The listing builds one solid part. Answer for the finished solid, in the listing's coordinates (mm). A direction names the side the tool comes from. Coordinates: 2 decimals unless noted, no trailing zeros. Order: outer loops, then holes, each group sorted by start corner. A loop starts at its lowest first (then second) coordinate and runs counter-clockwise, first axis right, second up.
```python
from build123d import *

# Parameters (mm, degrees)
BOSS_EXTRUDE1_DEPTH = 25
SKETCH2_R           = 11.025
CUT_EXTRUDE1_DEPTH  = 7
CUT_EXTRUDE3_DEPTH  = 8.75
CUT_EXTRUDE5_DEPTH  = 8.75
SKETCH5_R           = 1
CUT_EXTRUDE6_DEPTH  = 7.5
SKETCH6_R           = 1.95
CUT_EXTRUDE7_DEPTH  = 6.5
SKETCH7_R           = 2
CUT_EXTRUDE8_DEPTH  = 1
CUT_EXTRUDE9_DEPTH  = 62.065538563
CUT_EXTRUDE10_DEPTH = 3.5
SKETCH10_W          = 40
SKETCH10_H          = 5.05
CUT_EXTRUDE11_DEPTH = 7


with BuildPart() as part:
    # Sketch1 → Boss-Extrude1 (new body)
    with BuildSketch(Plane(origin=(0, 0, 0), x_dir=(1, 0, 0), z_dir=(0, 1, 0))):
        with BuildLine():
            Line((-42, -10), (42, -10))
            ThreePointArc((42, -10), (52, 0), (42, 10))
            Line((42, 10), (-42, 10))
            ThreePointArc((-42, 10), (-52, 0), (-42, -10))
        make_face()
    extrude(amount=BOSS_EXTRUDE1_DEPTH)

    # Sketch2 → Cut-Extrude1 (cut)
    with BuildSketch(Plane.XY.offset(10)):
        with Locations((0, 12.5)):
            Circle(SKETCH2_R)
    extrude(amount=-CUT_EXTRUDE1_DEPTH, mode=Mode.SUBTRACT)

    # Sketch3 → Cut-Extrude3 (cut)
    with BuildSketch(Plane.XZ):
        with BuildLine():
            Line((15, -10), (15, 10))
            Line((15, 10), (42, 10))
            ThreePointArc((42, 10), (52, 0), (42, -10))
            Line((42, -10), (15, -10))
        make_face()
        with BuildLine():
            Line((-15, -10), (-15, 10))
            Line((-15, 10), (-42, 10))
            ThreePointArc((-42, 10), (-52, 0), (-42, -10))
            Line((-42, -10), (-15, -10))
        make_face()
    extrude(amount=-CUT_EXTRUDE3_DEPTH, mode=Mode.SUBTRACT)

    # Sketch4 → Cut-Extrude5 (cut)
    with BuildSketch(Plane(origin=(0, 25, 0), x_dir=(1, 0, 0), z_dir=(0, 1, 0))):
        with BuildLine():
            Line((15, -10), (15, 10))
            Line((15, 10), (55, 10))
            ThreePointArc((55, 10), (65, 0), (55, -10))
            Line((55, -10), (15, -10))
        make_face()
        with BuildLine():
            Line((-15, -10), (-15, 10))
            Line((-15, 10), (-55, 10))
            ThreePointArc((-55, 10), (-65, 0), (-55, -10))
            Line((-55, -10), (-15, -10))
        make_face()
    extrude(amount=-CUT_EXTRUDE5_DEPTH, mode=Mode.SUBTRACT)

    # Sketch5 → Cut-Extrude6 (cut)
    with BuildSketch(Plane(origin=(0, 16.25, 0), x_dir=(1, 0, 0), z_dir=(0, 1, 0))):
        with Locations(Location((-42, 6.2, 0), (0, 0, 270))):
            Circle(SKETCH5_R)
        with Locations(Location((-35.8, 0, 0), (0, 0, 270))):
            Circle(SKETCH5_R)
        with Locations(Location((-42, -6.2, 0), (0, 0, 270))):
            Circle(SKETCH5_R)
        with Locations(Location((-48.2, 0, 0), (0, 0, 270))):
            Circle(SKETCH5_R)
        with Locations(Location((42, 6.2, 0), (0, 0, 270))):
            Circle(SKETCH5_R)
        with Locations(Location((48.2, 0, 0), (0, 0, 270))):
            Circle(SKETCH5_R)
        with Locations(Location((42, -6.2, 0), (0, 0, 270))):
            Circle(SKETCH5_R)
        with Locations(Location((35.8, 0, 0), (0, 0, 270))):
            Circle(SKETCH5_R)
    extrude(amount=-CUT_EXTRUDE6_DEPTH, mode=Mode.SUBTRACT)

    # Sketch6 → Cut-Extrude7 (cut)
    with BuildSketch(Plane.XZ.offset(-8.75)):
        with Locations(Location((-42, 6.2, 0), (0, 0, 270))):
            Circle(SKETCH6_R)
        with Locations(Location((-35.8, 0, 0), (0, 0, 270))):
            Circle(SKETCH6_R)
        with Locations(Location((-48.2, 0, 0), (0, 0, 270))):
            Circle(SKETCH6_R)
        with Locations(Location((-42, -6.2, 0), (0, 0, 270))):
            Circle(SKETCH6_R)
        with Locations(Location((42, 6.2, 0), (0, 0, 270))):
            Circle(SKETCH6_R)
        with Locations(Location((48.2, 0, 0), (0, 0, 270))):
            Circle(SKETCH6_R)
        with Locations(Location((35.8, 0, 0), (0, 0, 270))):
            Circle(SKETCH6_R)
        with Locations(Location((42, -6.2, 0), (0, 0, 270))):
            Circle(SKETCH6_R)
    extrude(amount=-CUT_EXTRUDE7_DEPTH, mode=Mode.SUBTRACT)

    # Sketch7 → Cut-Extrude8 (cut)
    with BuildSketch(Plane(origin=(0, 16.25, 0), x_dir=(1, 0, 0), z_dir=(0, 1, 0))):
        with Locations(Location((-42, 0, 0), (0, 0, 270))):
            Circle(SKETCH7_R)
        with Locations(Location((42, 0, 0), (0, 0, 270))):
            Circle(SKETCH7_R)
    extrude(amount=-CUT_EXTRUDE8_DEPTH, mode=Mode.SUBTRACT)

    # Sketch8 → Cut-Extrude9 (cut, through all)
    with BuildSketch(Plane.XY.offset(10)):
        with BuildLine():
            Line((-15, 16.25), (-15, 25))
            Line((-15, 25), (-9.100137362, 25))
            ThreePointArc((-9.100137362, 25), (-12.819702813, 21.143941218), (-15, 16.25))
        make_face()
        with BuildLine():
            Line((15, 0), (9.100137362, 0))
            ThreePointArc((9.100137362, 0), (12.819702813, 3.856058782), (15, 8.75))
            Line((15, 8.75), (15, 0))
        make_face()
        with BuildLine():
            Line((15, 25), (9.100137362, 25))
            ThreePointArc((9.100137362, 25), (12.819702813, 21.143941218), (15, 16.25))
            Line((15, 16.25), (15, 25))
        make_face()
        with BuildLine():
            Line((-15, 0), (-15, 8.75))
            ThreePointArc((-15, 8.75), (-12.819702813, 3.856058782), (-9.100137362, 0))
            Line((-9.100137362, 0), (-15, 0))
        make_face()
    extrude(amount=-CUT_EXTRUDE9_DEPTH, mode=Mode.SUBTRACT)

    # Sketch9 → Cut-Extrude10 (cut)
    with BuildSketch(Plane.XY.offset(3)):
        with BuildLine():
            Line((0.5, 10), (0.5, 7.525062814))
            ThreePointArc((0.5, 7.525062814), (5, 12.5), (0.5, 17.474937186))
            Line((0.5, 17.474937186), (0.5, 15))
            Line((0.5, 15), (-0.5, 15))
            Line((-0.5, 15), (-0.5, 17.474937186))
            ThreePointArc((-0.5, 17.474937186), (-5, 12.5), (-0.5, 7.525062814))
            Line((-0.5, 7.525062814), (-0.5, 10))
            Line((-0.5, 10), (0.5, 10))
        make_face()
    extrude(amount=-CUT_EXTRUDE10_DEPTH, mode=Mode.SUBTRACT)

    # Sketch10 → Cut-Extrude11 (cut)
    with BuildSketch(Plane.XY.offset(10)):
        with Locations((0, 12.5)):
            Rectangle(SKETCH10_W, SKETCH10_H)
    extrude(amount=-CUT_EXTRUDE11_DEPTH, mode=Mode.SUBTRACT)


solid = part.part
```
1) Each of these flat-tipped pins is pushed along its axis until it touches: P1, Ø6, axis at x = -48.2, z = 0, coming from the -Y side; P2, Ø2, axis at y = 11.5, z = -3.5, coming from the -X side; P3, Ø1.5, axis at y = 11.5, z = 7, coming from the -X side. Where does it stop, or does it pass through?
2) A cutting plane is placed at C-C, the plane z = -6.2. Write down the section's boundary in (x, y).
3) For faces 5 (the cylindrical face through (52, 12, 0)), 6 (the cylindrical face through (-12.862, 3.919, 0.14)), 7 (the cylindrical face through (-0.207, 1.477, 6.549)), 8 (the cylindrical face through (-43.904, 11.954, 6.623)), 9 (the flat face through (-42, 15.25, 0)), determine the directions among +Z, -Z, +X, -X, +Y, -Y from which every point of the face is accessible in a straight line to the end or side of a thin tool.
4) A cutting plane is placed at A-A, the plane x = 35.8. Write down the section's boundary in (y, z).
5) The mould has two halves that part along Y. Classify faces 1 (the cylindrical face through (5, 12.4, 1.3)), 2 (the flat face through (43, 15.25, 7)), 3 (the cylindrical face through (40, 16, 0)), 4 (the flat face through (0, 25, 0)): released by +Y, released by -Y, zero draft, split by the parting line, or undercut.
6) A cutting plane is placed at D-D, the plane z = 6.2. Count the separate pieces of the cut face and the enclosed holes in it, plus the area to 3 significant figures.
7) A cutting plane is placed at B-B, the plane x = 18. Write down the section's boundary in (y, z) (3 decimals), plus the area to 3 significant figures.
8) Straight lines are drawn through the part: probe 1 along X at (y, z) = (11.75, 6.2); probe 2 along X at (y, z) = (11.25, 7.25); probe 3 along X at (y, z) = (8.5, 2.75). For each, find the intervals that lie inside material, in ascending order.
Working result:
1. P1: stops at y = 8.75
1. P2: stops at x = -51.68
1. P3: stops at x = -49.81
2. outline: (-49.85, 8.75) - (-43.95, 8.75) - (-43.95, 15.25) - (-43, 15.25) - (-43, 16.25) - (-49.85, 16.25) - close; (-41, 15.25) - (-40.05, 15.25) - (-40.05, 8.75) - (-15, 8.75) arc R15.46 ccw to (-9.1, 0) - (9.1, 0) arc R15.46 ccw to (15, 8.75) - (40.05, 8.75) - (40.05, 15.25) - (41, 15.25) - (41, 16.25) - (15, 16.25) arc R15.46 ccw to (9.1, 25) - (-9.1, 25) arc R15.46 ccw to (-15, 16.25) - (-41, 16.25) - close; (43, 15.25) - (43.95, 15.25) - (43.95, 8.75) - (49.85, 8.75) - (49.85, 16.25) - (43, 16.25) - close
3. face 5: +X, +Y, -Y
3. face 6: +Z, -Z, -X, -Y
3. face 7: +Z
3. face 8: -Y
3. face 9: +Y
4. outline: (8.75, -10) - (16.25, -10) - (16.25, -1) - (15.25, -1) - (15.25, -1.95) - (8.75, -1.95) - close; (8.75, 1.95) - (15.25, 1.95) - (15.25, 1) - (16.25, 1) - (16.25, 10) - (8.75, 10) - close
5. face 1: undercut
5. face 2: released by -Y
5. face 3: zero draft
5. face 4: released by +Y
6. separate pieces: 3
6. enclosed holes: 1
6. area: 668 mm2
7. outline: (8.75, -10) - (16.25, -10) - (16.25, 10) - (15.025, 10) - (15.025, 3) - (9.975, 3) - (9.975, 10) - (8.75, 10) - close
7. area: 115 mm2
8. probe 1: x = -49.85 to -43.95, -40.05 to -20, 20 to 40.05, 43.95 to 49.85
8. probe 2: x = -48.89 to -43.64, -40.36 to -20, 20 to 40.36, 43.64 to 48.89
8. probe 3: x = -14.94 to -3, -0.5 to 0.5, 3 to 14.94
